Verification items for this drawing (mm, ordinates from the low corner). Round coordinates to 2 decimals unless told otherwise and drop trailing zeros. Write each loop counter-clockwise with the first axis right and the second up, starting at its lowest first coordinate (ties: lowest second). Pieces come first, ordered by that corner, then holes. Notation, with made-up numbers: (5, 24) -> (10, 24) arc R18 ccw to (10, 53) -> close; hole circle Ø3 at (1.25, 31). An arc over 180 degrees is marked (long way). Put each result on its own line as item: value. Start each with the question number.
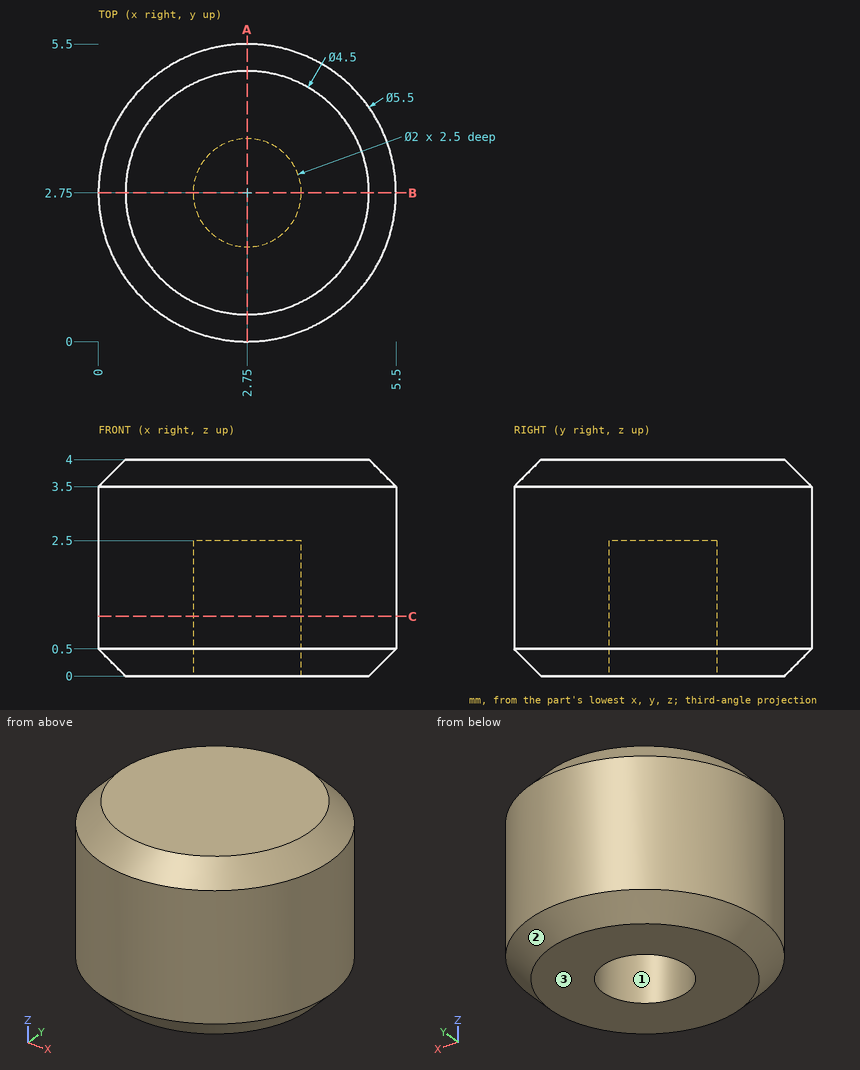
1. Material ranges on L1, parallel to Y at x = 2.75, z = 0.65; L2, parallel to Y at x = 3.35, z = 1.15; L3, parallel to X at y = 3.55, z = 2.4, recorded low to high. Write a range as [from, to].
2. Gauge pin test, flat ends, axial feed: P1, Ø2, axis at x = 3.5, y = 1, coming from the -Z side; P2, Ø1, axis at x = 3, y = 2.5, coming from the -Z side; P3, Ø1.5, axis at x = 1.5, z = 2, coming from the -Y side. Record the tip position at first contact, or that the pin passes through.
3. Section check A-A, the plane x = 2.75. Enter the section's corners in (y, z), then the cut area to 3 significant figures.
4. Section check C-C, the plane z = 1.1. Enter the section's corners in (x, y), then the cut area to 3 significant figures.
5. Draft check along X on the marked faces 1, 2 and 3. Enter one of: released by +X, released by -X, zero draft, split by the parting line, or undercut.
Reply:
1. L1: y = [0, 1.75], [3.75, 5.5]
1. L2: y = [0.07, 1.95], [3.55, 5.43]
1. L3: x = [0.12, 2.15], [3.35, 5.38]
2. P1: stops at z = 0
2. P2: stops at z = 2.5
2. P3: stops at y = 0.05
3. outline: (0, 0.5) -> (0.5, 0) -> (1.75, 0) -> (1.75, 2.5) -> (3.75, 2.5) -> (3.75, 0) -> (5, 0) -> (5.5, 0.5) -> (5.5, 3.5) -> (5, 4) -> (0.5, 4) -> (0, 3.5) -> close
3. area: 16.5 mm2
4. outline: circle Ø5.5 at (2.75, 2.75); hole circle Ø2 at (2.75, 2.75)
4. area: 20.6 mm2
5. face 1: undercut
5. face 2: split by the parting line
5. face 3: zero draft
